```python
from build123d import *

# Parameters (mm, degrees)
SCHIZZO2_R                   = 5
ESTRUSIONE_ESTRUSIONE1_DEPTH = 13
SCHIZZO3_R                   = 22
ESTRUSIONE_ESTRUSIONE2_DEPTH = 44


with BuildPart() as part:
    # Schizzo2 → Estrusione-Estrusione1 (new body)
    with BuildSketch(Plane.XY):
        with BuildLine():
            Line((-42.105263158, 12.334780679), (-7.894736842, 23.720732075))
            ThreePointArc((-7.894736842, 23.720732075), (0, 25), (7.894736842, 23.720732075))
            Line((7.894736842, 23.720732075), (42.105263158, 12.334780679))
            ThreePointArc((42.105263158, 12.334780679), (51, 0), (42.105263158, -12.334780679))
            Line((42.105263158, -12.334780679), (7.894736842, -23.720732075))
            ThreePointArc((7.894736842, -23.720732075), (0, -25), (-7.894736842, -23.720732075))
            Line((-7.894736842, -23.720732075), (-42.105263158, -12.334780679))
            ThreePointArc((-42.105263158, -12.334780679), (-51, 0), (-42.105263158, 12.334780679))
        make_face()
        with Locations((38, 0)):
            Circle(SCHIZZO2_R, mode=Mode.SUBTRACT)
        with Locations((-38, 0)):
            Circle(SCHIZZO2_R, mode=Mode.SUBTRACT)
    extrude(amount=-ESTRUSIONE_ESTRUSIONE1_DEPTH)

    # Schizzo3 → Estrusione-Estrusione2 (add)
    with BuildSketch(Plane.XY):
        Circle(SCHIZZO3_R)
    extrude(amount=ESTRUSIONE_ESTRUSIONE2_DEPTH)

    # Schizzo5 → Taglia-Rivoluzione2 (revolve, cut)
    with BuildSketch(Plane(origin=(0, 0, 0), x_dir=(1, 0, 0), z_dir=(0, 1, 0))):
        Polygon((0, 13), (-11, 13), (-11, -37.649147039), (-22, -44), (0, -44), align=None)
    revolve(axis=Axis((0, 0, -13), (0, 0, 1)), mode=Mode.SUBTRACT)


solid = part.part
```
Verification items for the finished model (mm, model axes). A direction names the side the tool comes from. Coordinates: 2 decimals unless noted, no trailing zeros. Write each loop counter-clockwise with the first axis right and the second up, starting at its lowest first coordinate (ties: lowest second). Pieces come first, ordered by that corner, then holes. Notation, with made-up numbers: (3, 8) - (31, 8) arc R30 ccw to (31, 39) - close; hole circle Ø2 at (-28.5, 75). An arc over 180 degrees is marked (long way). One line per question, with ' | ' between items. Start each with the question number.
1. Material ranges on line 1 along Y through (x, z) = (0.5, 25.5); line 2 along X through (y, z) = (0, 9.5); line 3 along Z through (x, y) = (-40, -12), recorded low to high.
2. Section check B-B (y = 0). Enter the section's corners in (x, z).
3. Draft check along X on faces 1 (the cylindrical face through (2.38, 10.74, 12.68)), 2 (the flat face through (25.239, -17.948, -6.409)), 3 (the cylindrical face through (0, 25, -6)). Enter one of: released by +X, released by -X, zero draft, split by the parting line, or undercut.
4. Access from +Z, -Z, +X, -X, +Y, -Y to the whole of each face (thin tool, end or side, straight path). Record for faces 4 (the cylindrical face through (33, 0, -6)), 5 (the flat face through (-22, -5, 0)).
5. Section check A-A (x = 0). Enter the section's corners in (y, z), plus the area to 3 significant figures.
6. Gauge pin test, flat ends, axial feed: P1, Ø12, axis at x = -24.5, z = 11, coming from the +Y side; P2, Ø8, axis at x = 38, y = 0, coming from the -Z side; P3, Ø1.5, axis at x = 10.5, z = -7, coming from the -Y side; P4, Ø12, axis at y = 2.5, z = 22, coming from the +X side. Record the tip position at first contact, or that the pin passes through.
7. Section check D-D (z = 13.5). Enter the section's corners in (x, y), plus the area to 3 significant figures.
8. Section check C-C (z = -3.5). Enter the section's corners in (x, y), plus the area to 3 significant figures.
Computed values:
1) line 1: -21.99 to -10.99, 10.99 to 21.99 | line 2: -22 to -11, 11 to 22 | line 3: -13 to 0
2) outline: (-51, -13) - (-43, -13) - (-43, 0) - (-51, 0) - close; (-33, -13) - (-11, -13) - (-11, 37.65) - (-22, 44) - (-22, 0) - (-33, 0) - close; (11, -13) - (33, -13) - (33, 0) - (22, 0) - (22, 44) - (11, 37.65) - close; (43, -13) - (51, -13) - (51, 0) - (43, 0) - close
3) face 1: undercut | face 2: released by +X | face 3: split by the parting line
4) face 4: +Z, -Z | face 5: +Z
5) outline: (-25, -13) - (-11, -13) - (-11, 37.65) - (-22, 44) - (-22, 0) - (-25, 0) - close; (11, -13) - (25, -13) - (25, 0) - (22, 0) - (22, 44) - (11, 37.65) - close | area: 1,260 mm²
6) P1: y = 11.91 | P2: through | P3: y = -23.1 | P4: x = 22
7) outline: circle Ø44 at (0, 0); hole circle Ø22 at (0, 0) | area: 1,140 mm²
8) outline: (-42.11, -12.33) - (-7.89, -23.72) arc R25 ccw to (7.89, -23.72) - (42.11, -12.33) arc R13 ccw to (42.11, 12.33) - (7.89, 23.72) arc R25 ccw to (-7.89, 23.72) - (-42.11, 12.33) arc R13 ccw to start; hole circle Ø10 at (-38, 0); hole circle Ø22 at (0, 0); hole circle Ø10 at (38, 0) | area: 3,030 mm²
